CAD build for the part. Positions are in the model's coordinates, mm. Give positions to 0.01 mm unless a question says otherwise; leave off trailing zeros. Order: outer loops, then holes, each group sorted by start corner. A loop starts at its lowest first (then second) coordinate and runs counter-clockwise, first axis right, second up. Notation, with made-up numbers: (86.5, -23.75) -> (131.5, -23.75) arc R19 ccw to (131.5, -12.75) -> close; hole circle Ø5 at (-28.5, 70). An arc over 180 degrees is marked (long way). Use one line per item in the form item = value. Start each with the question number.
1) Drop flat-ended pins along their axis: P1, Ø15, axis at x = 0, z = 0, coming from the -Y side; P2, Ø1, axis at x = -10, y = -0.5, coming from the -Z side. Give the stop position or say it passes through.
2) Cut at A-A, the plane x = -11.5. Give the cut face in (y, z).
3) Cut at B-B, the plane z = -12.5. Give the cut face in (x, y).
4) Probe line 1 (Y direction, x = 3.5, z = 8.5); line 2 (Z direction, x = 0, y = -0.8) (3 decimals); line 3 (Z direction, x = 0.5, y = -0.15). List the from-to ranges inside material, lowest first.
5) Mould opens along X. For faces 1 (the face through (0, 0, 0)), 2 (the face through (-7, -1, -7)) say: pulls with the +X half, pulls with the -X half, needs draft (parallel to the pull), parting line crosses it, or undercut.
from build123d import *

# Parameters (mm, degrees)
SKETCH1_R           = 15.875
BOSS_EXTRUDE1_DEPTH = 1
BOSS_EXTRUDE3_START = 1
SKETCH6_R           = 15.875
SKETCH6_R_2         = 9.525
BOSS_EXTRUDE3_DEPTH = 1
THREAD1_PITCH       = 0.25


with BuildPart() as part:
    # Sketch1 → Boss-Extrude1 (new body)
    with BuildSketch(Plane(origin=(0, 0, 0), x_dir=(1, 0, 0), z_dir=(0, 1, 0))):
        with Locations(Location((0, 0, 0), (0, 0, 270))):
            Circle(SKETCH1_R)
    extrude(amount=BOSS_EXTRUDE1_DEPTH)

    # Sketch6 → Boss-Extrude3 (add)
    with BuildSketch(Plane.XZ.offset(BOSS_EXTRUDE3_START)):
        with Locations(Location((0, 0, 0), (0, 0, 270))):
            Circle(SKETCH6_R)
        with Locations(Location((0, 0, 0), (0, 0, 270))):
            Circle(SKETCH6_R_2, mode=Mode.SUBTRACT)
    extrude(amount=-BOSS_EXTRUDE3_DEPTH)

    # Thread1: the profile of Thread Profile1 profile screwed along a right-hand helix of 4 turns, 6 arcs to a turn; built about Z, then put on its axis
    thread1_z = Axis((0, 0, 0), (0, 0, 1))
    thread1_corners = [(9.5247, 0, -0.000173205), (9.660316469, 0, 0.078125), (9.660316469, 0, 0.109375), (9.5247, 0, 0.187673204)]
    with BuildLine(mode=Mode.PRIVATE) as thread1_profile:
        Line(thread1_corners[0], thread1_corners[1])
        Line(thread1_corners[1], thread1_corners[2])
        Line(thread1_corners[2], thread1_corners[3])
        Line(thread1_corners[3], thread1_corners[0])
    thread1_cap = Face(thread1_profile.wire())
    thread1_turn_angles = [0, 30, 60, 90, 120, 150, 180, 210, 240, 270, 300, 330, 360]
    thread1_turn_weights = [1, 0.8660254037844387, 1, 0.8660254037844387, 1, 0.8660254037844387, 1, 0.8660254037844387, 1, 0.8660254037844387, 1, 0.8660254037844387, 1]
    thread1_turn_rails = [Edge.make_bspline([Vector(p[0], p[1], 0).rotate(thread1_z, thread1_turn_angles[k]) / thread1_turn_weights[k] + Vector(0, 0, p[2] + THREAD1_PITCH * thread1_turn_angles[k] / 360) for k in range(13)], [0, 0, 0, 1, 1, 2, 2, 3, 3, 4, 4, 5, 5, 6, 6, 6], 2, thread1_turn_weights) for p in thread1_corners]
    thread1_turn_sides = [Face.make_surface_from_curves(thread1_turn_rails[p[0]], thread1_turn_rails[p[1]]) for p in [(0, 1), (1, 2), (2, 3), (3, 0)]]
    thread1 = Plane(origin=(0, -1, 0), x_dir=(1, 0, 0), z_dir=(0, 1, 0)) * Solid(Shell([*[p.moved(Location((0, 0, THREAD1_PITCH * i))) for i in range(4) for p in thread1_turn_sides], thread1_cap, thread1_cap.rotate(thread1_z, 1440).moved(Location((0, 0, THREAD1_PITCH * 1440 / 360)))]))
    add(thread1, mode=Mode.SUBTRACT)


solid = part.part
Result:
q1.P1 = 0
q1.P2 = -12.72
q2.outline = (-1, -10.94) -> (1, -10.94) -> (1, 10.94) -> (-1, 10.94) -> close
q3.outline = (-9.79, -1) -> (9.79, -1) -> (9.79, 1) -> (-9.79, 1) -> close
q4.line_1 = 0 to 1
q4.line_2 = -15.875 to -9.612, 9.547 to 15.875
q4.line_3 = -15.87 to -9.58, 9.56 to 15.87
q5.face_1 = undercut
q5.face_2 = needs draft
